The drawing under review shows one solid part. Ordinate dimensions are in mm from its lowest x, y, z. A direction names the side the tool comes from. Coordinates: 2 decimals unless noted, no trailing zeros. Order: outer loops, then holes, each group sorted by start corner. A loop starts at its lowest first (then second) coordinate and runs counter-clockwise, first axis right, second up.
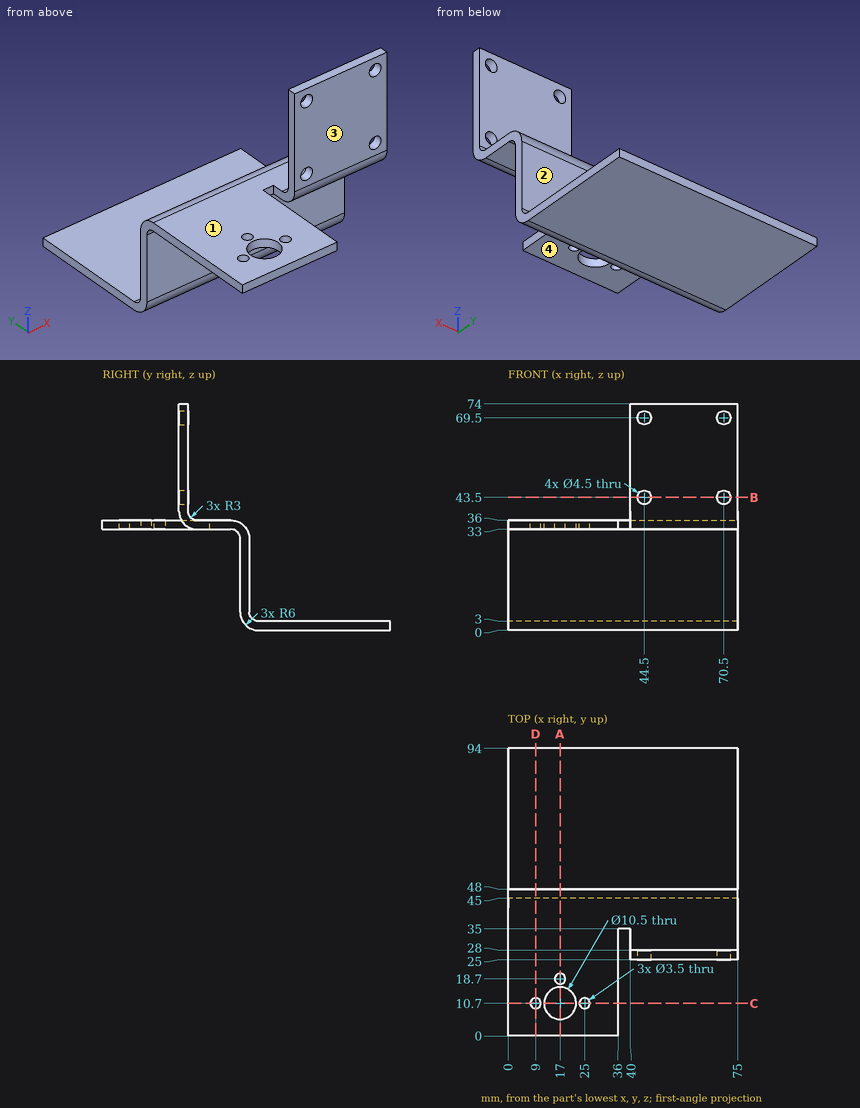
(1) Machinability: for the marked faces 1, 2, 3 and 4, which of the approach directions +Z, -Z, +X, -X, +Y, -Y give a long, thin tool a straight path to every point of the face, cutting with its end or side? Answer none if there is none.
A:
face 1: +Z, -X, +Y
face 2: +Z, +X, -X, +Y
face 3: +Z, -Z, +X, -X, -Y
face 4: -Z, +X, -X, -Y
(2) Wall thickness on probe 1 along X at (y, z) = (10.7, 34.25); probe 2 along X at (y, z) = (10, 34); probe 3 along Z at (x, y) = (70.5, 27.35): over which ranges is each line inside the solid? List them lowest first.
A:
probe 1: x = 0 to 7.25, 10.75 to 11.75, 22.25 to 23.25, 26.75 to 36
probe 2: x = 0 to 7.4, 10.6 to 11.8, 22.2 to 23.4, 26.6 to 36
probe 3: z = 34.24 to 41.25, 45.75 to 67.25, 71.75 to 74
(3) We need section D-D, the plane x = 9. Write out the cut boundary in (y, z), and give its area (3 significant figures).
A:
outline: (0, 33) - (8.95, 33) - (8.95, 36) - (0, 36) - close; (12.45, 33) - (42, 33) arc R3 cw to (45, 30) - (45, 6) arc R6 ccw to (51, 0) - (94, 0) - (94, 3) - (51, 3) arc R3 cw to (48, 6) - (48, 30) arc R6 ccw to (42, 36) - (12.45, 36) - close
area: 359 mm2
(4) We need section A-A, the plane x = 17. Write out the cut boundary in (y, z).
A:
outline: (0, 33) - (5.45, 33) - (5.45, 36) - (0, 36) - close; (15.95, 33) - (16.95, 33) - (16.95, 36) - (15.95, 36) - close; (20.45, 33) - (42, 33) arc R3 cw to (45, 30) - (45, 6) arc R6 ccw to (51, 0) - (94, 0) - (94, 3) - (51, 3) arc R3 cw to (48, 6) - (48, 30) arc R6 ccw to (42, 36) - (20.45, 36) - close
(5) For pin 1 Ø6 at (x, z) = (44.5, 43.5) entering from -Y; pin 2 Ø8 at (x, z) = (18, 28.5) entering from +Y; pin 3 Ø4 at (x, y) = (9, 10.7) entering from -Z, all flat-tipped, find the tip position at first contact; note any pin that passes through.
A:
pin 1: stops at y = 25
pin 2: stops at y = 48
pin 3: stops at z = 33
(6) We need section C-C, the plane y = 10.7. Write out the cut boundary in (x, z).
A:
outline: (0, 33) - (7.25, 33) - (7.25, 36) - (0, 36) - close; (10.75, 33) - (11.75, 33) - (11.75, 36) - (10.75, 36) - close; (22.25, 33) - (23.25, 33) - (23.25, 36) - (22.25, 36) - close; (26.75, 33) - (36, 33) - (36, 36) - (26.75, 36) - close
(7) We need section B-B, the plane z = 43.5. Write out the cut boundary in (x, y).
A:
outline: (40, 25) - (42.25, 25) - (42.25, 28) - (40, 28) - close; (46.75, 25) - (68.25, 25) - (68.25, 28) - (46.75, 28) - close; (72.75, 25) - (75, 25) - (75, 28) - (72.75, 28) - close
